Geometry: final body of the model. Coordinates: model frame, mm. A direction names the side the tool comes from. Give positions to 0.01 mm unless a question says otherwise; leave off trailing zeros. Write each loop counter-clockwise with the first axis right and the second up, starting at its lowest first coordinate (ties: lowest second). Pieces come first, ordered by that corner, then holes.
Q1. Reachability of faces 1 (the cylindrical face through (165.155, -25.7, -3.859)), 2 (the cylindrical face through (102.894, -18.609, -2.465)) from +Z, -Z, +X, -X, +Y, -Y: full face, straight path, thin tool, end or side. Return the list, or none.
Q2. Line query: line 1 (X direction, y = -20, z = -1.05); line 2 (Y direction, x = 172, z = -4.7); line 3 (X direction, y = -16, z = -3.3). Output: solid intervals per line, ascending.
Q3. Pin query (flat end, axial travel): pin 1 Ø3.5 at (x, y) = (114, -21) entering from -Z; pin 2 Ø1.5 at (y, z) = (-15.5, -4) entering from -X; pin 3 Ø13 at (x, y) = (174, -20) entering from -Z. Return the tip coordinate at first contact, or that it passes through.
Q4. Mould query, pull axis X, two halves, no side actions, for faces 3 (the cylindrical face through (176.94, -14.88, -1.21)), 4 (the flat face through (140, -21, -5)), 5 (the cylindrical face through (173.27, -20.29, -0.99)), 6 (the cylindrical face through (115.814, -18.127, -2.028)). Classes: +X half, -X half, draft (parallel to the pull), parting line (faces both ways), or undercut.
Q5. Section C-C (x = 139.5). Return the cut outline in (y, z), plus the area to 3 significant figures.
Q6. Section D-D (y = -30). Return the cut outline in (x, z).
Q7. Section A-A (y = -19). State how many separate pieces and enclosed holes the cut face has, plus the area to 3 significant figures.
Q8. Section B-B (y = -24). Return the cut outline in (x, z), plus the area to 3 significant figures.
Autodesk Inventor part; units mm, degrees
ref_plane "YZ Plane" through (0, 0, 0) normal (1, 0, 0) x (0, 1, 0)
ref_plane "XZ Plane" through (0, 0, 0) normal (0, 1, 0) x (-1, 0, 0)
ref_plane "XY Plane" through (0, 0, 0) normal (0, 0, 1) x (1, 0, 0)
sketch "スケッチ1" plane through (0, 0, 0) normal (0, 0, 1) x (1, 0, 0)
  line L0 (-101.5, 48) -> (108.5, 48)
  circle A0 centre (111.885, -19) radius 4
  circle A1 centre (171.8807, -19.7195) radius 4
  circle A2 centre (111.885, -19) radius 7
  circle A3 centre (171.8807, -19.7195) radius 7
  line L1 (171.8807, -19.7195) -> (111.885, -19) construction
  line L2 (171.9647, -12.72) -> (111.969, -12.0005)
  line L3 (111.8011, -25.9995) -> (171.7968, -26.719)
  arc A4 (171.7968, -26.719) -> (171.9647, -12.72) centre (171.8807, -19.7195) ccw
  arc A5 (111.969, -12.0005) -> (111.8011, -25.9995) centre (111.885, -19) ccw
  line L4 (173.7961, -12.9866) -> (250.1906, -34.7195)
  circle A6 centre (241.9819, -63.5746) radius 30
  line L5 (268.18, -78.1916) -> (221.9512, -41.2414)
  line L6 (221.9512, -41.2414) -> (169.9654, -26.4523)
  line L7 (271.9819, -113.1361) -> (271.9819, -54.8199)
  line L8 (111.885, -19) -> (111.885, 41) construction
  line L9 (118.885, -19) -> (118.885, 41)
  line L10 (104.885, 41) -> (104.885, -19)
  arc A7 (104.885, -19) -> (118.885, -19) centre (111.885, -19) ccw
  arc A8 (118.885, 41) -> (104.885, 41) centre (111.885, 41) ccw
  circle A9 centre (29.4318, 47.238) radius 30
  line L11 (113.3193, 34.1485) -> (35.5787, 17.8745)
  line L12 (-0.5585, 48) -> (57.5489, 36.7771)
  line L13 (57.5489, 36.7771) -> (110.4508, 47.8515)
  circle A10 centre (113.5, -20) radius 68
  line L14 (321.9635, -82.9551) -> (60.2705, 100.2843)
  line L15 (259.1892, -39) -> (111.885, -19)
  arc A11 (93.5924, -27.1048) -> (135.371, -5.9244) centre (95.0604, 21.7941) ccw
  arc A12 (135.371, -5.9244) -> (135.8476, -3.6716) centre (132.899, -4.2246) ccw
  arc A13 (135.8476, -3.6716) -> (83.1833, 18.5565) centre (102.1579, -9.9896) ccw
  line L16 (111.885, -19) -> (112.6892, 40.9946) construction
  line L17 (118.8844, -19.0938) -> (119.6886, 40.9008)
  line L18 (105.6898, 41.0884) -> (104.8857, -18.9062)
  arc A14 (104.8857, -18.9062) -> (118.8844, -19.0938) centre (111.885, -19) ccw
  arc A15 (119.6886, 40.9008) -> (105.6898, 41.0884) centre (112.6892, 40.9946) ccw
  line L19 (164.9949, 48) -> (164.9949, 26)
  line L20 (164.9949, 26) -> (327.4949, -102)
  circle A16 centre (116.2926, -40) radius 68
  circle A17 centre (-98.885, 0) radius 67.5
  line L21 (321.3633, -8.501) -> (-152.6681, 78.4982)
  line L22 (104.8897, -3) -> (104.8897, 0)
  line L23 (104.8897, -3) -> (72.0656, -3)
  line L24 (72.0656, 0) -> (104.8897, 0)
  circle A18 centre (83.3769, -17.5) radius 13.85
  line L25 (178.7705, -28.9572) -> (174.2123, -32.8589)
  line L26 (174.2123, -32.8589) -> (164.8807, -30.2042)
  line L27 (164.8807, -30.2042) -> (164.8807, -19.7195)
  line L28 (169.9654, -26.4523) -> (168.5972, -31.2615)
  line L29 (168.5972, -31.2615) -> (164.8807, -26.636)
  line L30 (178.8802, -19.8034) -> (178.6547, -38.6089)
  line L31 (165.0125, -21.0715) -> (158.1724, 13.6763)
  circle A19 centre (171.8807, -19.7195) radius 7.5
  point P0 (0, 0)
  point P1 (141.8829, -19.3597)
  point P2 (111.885, 11)
  point P3 (105.885, 0)
  point P4 (105.885, 0)
  point P5 (23.7328, -42.729)
  point P6 (112.2871, 10.9973)
  point P7 (169.2723, -12.6877)
  point P8 (163.3482, -12.6166)
  point P9 (164.4925, -18.4296)
  point P10 (172.5552, -27.1891)
  point P11 (178.8479, -22.4958)
  dimension "d0" = 8
  dimension "d1" = 8
  dimension "d2" = 3
  dimension "d3" = 3
  dimension "d4" = 60
  dimension "d5" = 14
  dimension "d6" = 14
  dimension "d7" = 60
  dimension "d8" = 14
  dimension "d9" = 60
  dimension "d10" = 14
  dimension "d11" = 6
  dimension "d12" = 35
  dimension "d13" = 13.271
  dimension "d14" = 14
  dimension "d15" = 20
  dimension "d16" = 15
  dimension "d17" = 22
  dimension "d18" = 150
  dimension "d19" = 162.5
  dimension "d20" = 0
  dimension "d21" = 136
  dimension "d22" = 136
  dimension "d23" = 135
  dimension "d24" = 38.227
  dimension "d25" = 18
  dimension "d27" = 5
  dimension "d28" = 6
  dimension "d30" = 101.823
  dimension "d31" = 101.823
  dimension "d32" = 0.5
extrude "押し出し1" add sketch "スケッチ1" against normal blind 5 contours L25 L26 L28 A19 L15 L6 | L6 L15 L30 | L15 A19 L6 | L6 A19 L30 L15 | A19 L15 L28 L3 L6 | L6 L3 A3 L30 A19 | A19 L28 L15 | L29 L3 L15 A19 L28 | L26 L27 L29 | A2 A11 | L6 A3 L3 | L3 L28 L6 | L28 A19 L15 | L15 A19 L3 L28 | L27 L15 L3 | L3 A2 A11 L15 L27 | A3 | L9 A2 L2 | L2 L17 L9 | L3 A19 L27 L31 A3 L28 | L15 L3 A19 | A2 A11 | L15 L27 A19 L3 | L15 A11 L2 L31 A19 L27 | A19 L31 L2 | L2 A3 L27 L31 A19 | L2 A11 L15 A2 L17 | L31 L27 A3 | A2 L15 A11 | A19 L31 L27 | A0 | A1
extrude "押し出し2" cut sketch "スケッチ1" against normal blind 2.75 contours L6 L15 L30 | L6 A19 L30 L15 | A19 L15 L28 L3 L6 | L6 L3 A3 L30 A19 | A19 L28 L15 | L30 A3 L4 A19 | L6 A3 L3 | L3 L28 L6 | L28 A19 L15 | L15 A19 L3 L28 | A3 | L4 A3 L2 A19 | L3 A19 L27 L31 A3 L28 | A19 L31 L2 | L2 A3 L27 L31 A19 | L31 L27 A3 | A19 L31 L27 | A1
hole "穴1" at (105.885, 0, 0) at (23.7328, -42.729, 0) at (116.2926, -40, 0) at (-98.885, 0, 0) at (171.8807, -19.7195, 0) direction (0, 0, -1) diameter 3 depth 12 tip angle 118
sketch "スケッチ2" plane through (0, 0, 0) normal (0, 0, 1) x (1, 0, 0)
  line L0 (163.3482, -12.6166) -> (164.4925, -18.4296)
  arc A0 (164.4925, -18.4296) -> (172.5552, -27.1891) centre (171.8807, -19.7195) ccw
  line L1 (172.5552, -27.1891) -> (178.7705, -28.9572)
  line L2 (178.7705, -28.9572) -> (174.2123, -32.8589)
  line L3 (174.2123, -32.8589) -> (164.8807, -30.2042)
  line L4 (164.8807, -30.2042) -> (164.8807, -26.636)
  line L5 (164.8807, -26.636) -> (111.8011, -25.9995)
  arc A1 (111.969, -12.0005) -> (111.8011, -25.9995) centre (111.885, -19) ccw
  line L6 (111.969, -12.0005) -> (163.3482, -12.6166)
  circle A2 centre (171.8807, -19.7195) radius 7.5
  circle A3 centre (171.8807, -19.7195) radius 12.5
  point P0 (0, 0)
  point P1 (161.4414, -26.5948)
  point P2 (164.8807, -30.0756)
  point P3 (165.2308, -30.3038)
  point P4 (171.9637, -32.2192)
  dimension "d44" = 5
extrude "押し出し3" add sketch "スケッチ2" against normal blind 5 contours L5 L4 A3 | A3 L3
sketch "スケッチ3" plane through (0, 0, 0) normal (0, 0, 1) x (1, 0, 0)
  line L0 (163.3482, -12.6166) -> (164.4925, -18.4296)
  arc A0 (164.4925, -18.4296) -> (172.5552, -27.1891) centre (171.8807, -19.7195) ccw
  line L1 (172.5552, -27.1891) -> (178.7705, -28.9572)
  line L2 (178.7705, -28.9572) -> (174.2123, -32.8589)
  line L3 (174.2123, -32.8589) -> (171.9637, -32.2192)
  arc A1 (165.2308, -30.3038) -> (171.9637, -32.2192) centre (171.8807, -19.7195) ccw
  line L4 (165.2308, -30.3038) -> (164.8807, -30.2042)
  line L5 (164.8807, -30.2042) -> (164.8807, -30.0756)
  arc A2 (161.4414, -26.5948) -> (164.8807, -30.0756) centre (171.8807, -19.7195) ccw
  line L6 (161.4414, -26.5948) -> (111.8011, -25.9995)
  arc A3 (111.969, -12.0005) -> (111.8011, -25.9995) centre (111.885, -19) ccw
  line L7 (111.969, -12.0005) -> (163.3482, -12.6166)
  circle A4 centre (171.8807, -19.7195) radius 12.5
  point P0 (0, 0)
  point P1 (165.2308, -30.3038)
extrude "押し出し4" cut sketch "スケッチ3" against normal blind 10 contours A4 L4 L5
hole "穴2" at (105.885, 0, 0) at (111.885, -19, 0) direction (0, 0, -1) diameter 8.05 depth 12 tip angle 118
sketch "スケッチ4" plane through (0, 0, 0) normal (0, 0, 1) x (1, 0, 0)
  circle A0 centre (111.885, -19) radius 4.025
  line L0 (163.3482, -12.6166) -> (164.4925, -18.4296)
  arc A1 (164.4925, -18.4296) -> (172.5552, -27.1891) centre (171.8807, -19.7195) ccw
  line L1 (172.5552, -27.1891) -> (178.7705, -28.9572)
  line L2 (178.7705, -28.9572) -> (174.2123, -32.8589)
  line L3 (174.2123, -32.8589) -> (171.9637, -32.2192)
  arc A2 (161.4414, -26.5948) -> (171.9637, -32.2192) centre (171.8807, -19.7195) ccw
  line L4 (161.4414, -26.5948) -> (111.8011, -25.9995)
  arc A3 (111.969, -12.0005) -> (111.8011, -25.9995) centre (111.885, -19) ccw
  line L5 (111.969, -12.0005) -> (163.3482, -12.6166)
  arc A4 (164.4925, -18.4296) -> (172.5552, -27.1891) centre (171.8807, -19.7195) ccw
  circle A5 centre (171.8807, -19.7195) radius 7.5
  circle A6 centre (171.8807, -19.7195) radius 9
  line L6 (178.7705, -28.9572) -> (172.5552, -27.1891)
  line L7 (164.4925, -18.4296) -> (163.3482, -12.6166)
  circle A7 centre (111.885, -19) radius 9
  point P0 (0, 0)
  point P1 (175.4063, -28.0002)
  point P2 (163.9203, -15.5231)
  point P3 (163.92, -15.5211)
  point P4 (175.4063, -28.0002)
  dimension "d56" = 15
  dimension "d57" = 1.5
  dimension "d58" = 18
extrude "押し出し5" add sketch "スケッチ4" against normal blind 5 contours A7 L4 A3 L5 | L5 A3 L4 A7
extrude "押し出し6" cut sketch "スケッチ4" against normal blind 2.75 contours L0 A1 L1 A6
sketch "スケッチ6" plane through (0, 0, 0) normal (0, 0, 1) x (1, 0, 0)
  circle A0 centre (171.8807, -19.7195) radius 1.5
  line L0 (163.3482, -12.6166) -> (171.9647, -12.72)
  line L1 (163.92, -15.5211) -> (163.3482, -12.6166)
  arc A1 (163.92, -15.5211) -> (175.4063, -28.0002) centre (171.8807, -19.7195) ccw
  line L2 (178.7705, -28.9572) -> (175.4063, -28.0002)
  line L3 (178.8802, -19.8034) -> (178.7705, -28.9572)
  arc A2 (178.8802, -19.8034) -> (171.9647, -12.72) centre (171.8807, -19.7195) ccw
  point P0 (0, 0)
extrude "押し出し8" cut sketch "スケッチ6" against normal blind 10
extrude "押し出し9" add sketch "スケッチ6" against normal blind 2.45
sketch "スケッチ7" plane through (0, 0, -5) normal (0, 0, -1) x (-1, 0, 0)
  arc A0 (-117.4576, -26.0673) -> (-117.6254, -12.0683) centre (-111.885, -19) ccw
  line L0 (-117.4576, -26.0673) -> (-161.4414, -26.5948)
  arc A1 (-171.9637, -32.2192) -> (-161.4414, -26.5948) centre (-171.8807, -19.7195) ccw
  line L1 (-171.9637, -32.2192) -> (-174.2123, -32.8589)
  line L2 (-174.2123, -32.8589) -> (-178.7705, -28.9572)
  line L3 (-178.7705, -28.9572) -> (-175.4063, -28.0002)
  arc A2 (-175.4063, -28.0002) -> (-163.92, -15.5211) centre (-171.8807, -19.7195) ccw
  line L4 (-163.92, -15.5211) -> (-163.3482, -12.6166)
  line L5 (-163.3482, -12.6166) -> (-117.6254, -12.0683)
  circle A3 centre (-111.885, -19) radius 4.025
  circle A4 centre (-111.885, -19) radius 6
  point P0 (0, 0)
  dimension "d70" = 12
extrude "押し出し10" cut sketch "スケッチ7" against normal blind 1 contours A4
sketch "スケッチ8" plane through (0, 0, -5) normal (0, 0, -1) x (-1, 0, 0)
  circle A0 centre (-111.885, -19) radius 6
  arc A1 (-117.4576, -26.0673) -> (-117.6254, -12.0683) centre (-111.885, -19) ccw
  line L0 (-117.4576, -26.0673) -> (-161.4414, -26.5948)
  arc A2 (-171.9637, -32.2192) -> (-161.4414, -26.5948) centre (-171.8807, -19.7195) ccw
  line L1 (-171.9637, -32.2192) -> (-174.2123, -32.8589)
  line L2 (-174.2123, -32.8589) -> (-178.7705, -28.9572)
  line L3 (-178.7705, -28.9572) -> (-175.4063, -28.0002)
  arc A3 (-175.4063, -28.0002) -> (-163.92, -15.5211) centre (-171.8807, -19.7195) ccw
  line L4 (-163.92, -15.5211) -> (-163.3482, -12.6166)
  line L5 (-163.3482, -12.6166) -> (-117.6254, -12.0683)
  circle A4 centre (-171.8807, -19.7195) radius 1.5
  circle A5 centre (-171.8807, -19.7195) radius 3
  point P0 (0, 0)
  dimension "d73" = 6
extrude "押し出し11" cut sketch "スケッチ8" against normal blind 3 contours A5
equation "\"d9\" = d7"
equation "\"d31\" = d30"
properties part number "後ろウィング中間(ミラー)"
Computed:
1. face 1: -Z
1. face 2: +Z, -Z
2. line 1: x = 102.94 to 107.99, 115.78 to 170.41, 173.35 to 178.88
2. line 2: y = -32.23 to -28.72
2. line 3: x = 103.4 to 109.2, 114.57 to 163.69
3. pin 1: stops at z = -4
3. pin 2: stops at x = 103.32
3. pin 3: stops at z = -2.45
4. face 3: +X half
4. face 4: draft
4. face 5: undercut
4. face 6: undercut
5. outline: (-26.33, -5) - (-12.33, -5) - (-12.33, 0) - (-26.33, 0) - close
5. area: 70.0 mm2
6. outline: (164.77, -5) - (177.55, -5) - (177.55, 0) - (164.77, 0) - close
7. separate pieces: 3
7. enclosed holes: 0
7. area: 287 mm2
8. outline: (104.4, -5) - (108.57, -5) - (108.57, -4) - (115.2, -4) - (115.2, -5) - (163.96, -5) - (163.96, -2.45) - (178.83, -2.45) - (178.83, 0) - (104.4, 0) - close
8. area: 328 mm2
